```python
from build123d import *

# Parameters (mm, degrees)
EXTRUDE_1_DEPTH                 = 60
SKETCH_3_W                      = 44.3
SKETCH_3_H                      = 33.8
CUT_EXTRUDE_1_DEPTH             = 56.5
SKETCH_4_W                      = 75
SKETCH_4_H                      = 30
EXTRUDE_2_DEPTH                 = 66
SKETCH_5_W                      = 59.221662283
SKETCH_5_H                      = 50
CUT_EXTRUDE_2_DEPTH             = 65
SKETCH_34_W                     = 75
SKETCH_34_H                     = 30
EXTRUDE_5_DEPTH                 = 0.5
HOLE_WIZARD_M3_1_AT_2_COUNT     = 2
HOLE_WIZARD_M3_1_AT_2_PITCH     = 21
HOLE_WIZARD_M3_1_AT_3_COUNT     = 2
HOLE_WIZARD_M3_1_AT_3_PITCH     = 24.186773245
HOLE_WIZARD_M3_1_AT_4_COUNT     = 2
HOLE_WIZARD_M3_1_AT_4_PITCH     = 12
SKETCH_9_W                      = 201.131722391
SKETCH_9_H                      = 182.70094424
CUT_EXTRUDE_3_DEPTH             = 10
SKETCH_10_W                     = 66.5
SKETCH_10_H                     = 50
CUT_EXTRUDE_4_DEPTH             = 1.2
HOLE_WIZARD_M2_5_1_D            = 2.7
HOLE_WIZARD_M2_5_1_CBORE_D      = 5.5
HOLE_WIZARD_M2_5_1_CBORE_DEPTH  = 2.9
EXTRUDE_3_DEPTH                 = 12
SKETCH_16_W                     = 66.5
SKETCH_16_H                     = 53.8
EXTRUDE_4_DEPTH                 = 3
HOLE_WIZARD_M2_5_2_D            = 2.7
HOLE_WIZARD_M2_5_2_DEPTH        = 10
HOLE_WIZARD_M2_5_2_CBORE_D      = 5.5
HOLE_WIZARD_M2_5_2_CBORE_DEPTH  = 5
HOLE_START                      = -61.2
HOLE_WIZARD_2_9_2_9_1_OUTLINE_R = 1.45
HOLE_WIZARD_2_9_2_9_1_DEPTH     = 10
HOLE_START_2                    = -56.2
HOLE_WIZARD_2_9_2_9_2_OUTLINE_R = 1.45
HOLE_WIZARD_2_9_2_9_2_DEPTH     = 5
HOLE_WIZARD_2_9_2_9_4_D         = 2.9
HOLE_WIZARD_2_9_2_9_4_DEPTH     = 7
HOLE_WIZARD_2_9_2_9_4_TIP       = 0.871247898
CUT_EXTRUDE_5_REACH             = 165.928


# Read off the part's stored shape, not the designer's step: Ø2.9 (2.9) 直径孔1, Ø2.9 (2.9) 直径孔2, Ø2.9 (2.9) 直径孔3
with BuildPart() as part:
    # 草图2 → 凸台-拉伸1 (new body)
    with BuildSketch(Plane.XY):
        Polygon((0, 0), (15.232865332, 0), (15.232865332, -50), (66.5, -50), (66.5, -105), (0, -105), align=None)
    extrude(amount=EXTRUDE_1_DEPTH)

    # 草图3 → 切除-拉伸1 (cut)
    with BuildSketch(Plane.ZY):
        with Locations((37.85, -78.1)):
            Rectangle(SKETCH_3_W, SKETCH_3_H)
    extrude(amount=-CUT_EXTRUDE_1_DEPTH, mode=Mode.SUBTRACT)

    # 草图4 → 凸台-拉伸2 (add)
    with BuildSketch(Plane.ZY):
        with Locations((37.5, -120)):
            Rectangle(SKETCH_4_W, SKETCH_4_H)
    extrude(amount=-EXTRUDE_2_DEPTH)

    # 草图5 → 切除-拉伸2 (cut)
    with BuildSketch(Plane.XY.offset(60)):
        with Locations((-14.37796581, -25)):
            Rectangle(SKETCH_5_W, SKETCH_5_H)
    extrude(amount=-CUT_EXTRUDE_2_DEPTH, mode=Mode.SUBTRACT)

    # 草图34 → 凸台-拉伸5 (add)
    with BuildSketch(Plane(origin=(66, 0, 0), x_dir=(0, 0, -1), z_dir=(1, 0, 0))):
        with Locations((-37.5, -120)):
            Rectangle(SKETCH_34_W, SKETCH_34_H)
    extrude(amount=EXTRUDE_5_DEPTH)

    # 草图8 → M3 六角凹头螺钉的柱形沉头孔1 (revolve, cut)
    with BuildSketch(Plane(origin=(66, -108.3, 54.5), x_dir=(0, 0, -1), z_dir=(0, 1, 0))):
        Polygon((0, 0), (0, 66), (1.45, 66), (1.45, 60), (3.25, 60), (3.25, 0), align=None)
    hole_wizard_m3_1 = revolve(axis=Axis((72.35, -108.3, 54.5), (-1, 0, 0)), mode=Mode.SUBTRACT)

    # M3 六角凹头螺钉的柱形沉头孔1 at 2: M3 六角凹头螺钉的柱形沉头孔1 ×2
    with Locations(*[(0, 0, -i * HOLE_WIZARD_M3_1_AT_2_PITCH) for i in range(1, HOLE_WIZARD_M3_1_AT_2_COUNT)]):
        add(hole_wizard_m3_1, mode=Mode.SUBTRACT)

    # M3 六角凹头螺钉的柱形沉头孔1 at 3: M3 六角凹头螺钉的柱形沉头孔1 ×2
    with Locations(*[Vector(0, -0.4961389383568334, -0.8682431421244595) * (i * HOLE_WIZARD_M3_1_AT_3_PITCH) for i in range(1, HOLE_WIZARD_M3_1_AT_3_COUNT)]):
        add(hole_wizard_m3_1, mode=Mode.SUBTRACT)

    # M3 六角凹头螺钉的柱形沉头孔1 at 4: M3 六角凹头螺钉的柱形沉头孔1 ×2
    with Locations(*[(0, -i * HOLE_WIZARD_M3_1_AT_4_PITCH, 0) for i in range(1, HOLE_WIZARD_M3_1_AT_4_COUNT)]):
        add(hole_wizard_m3_1, mode=Mode.SUBTRACT)

    # 草图9 → 切除-拉伸3 (cut)
    with BuildSketch(Plane(origin=(0, 0, 0), x_dir=(-1, 0, 0), z_dir=(0, 0, -1))):
        with Locations((-9.064738267, -112.548341422)):
            Rectangle(SKETCH_9_W, SKETCH_9_H)
    extrude(amount=-CUT_EXTRUDE_3_DEPTH, mode=Mode.SUBTRACT)

    # 草图10 → 切除-拉伸4 (cut)
    with BuildSketch(Plane(origin=(0, -50, 0), x_dir=(1, 0, 0), z_dir=(0, 1, 0))):
        with Locations((33.25, -35)):
            Rectangle(SKETCH_10_W, SKETCH_10_H)
    extrude(amount=-CUT_EXTRUDE_4_DEPTH, mode=Mode.SUBTRACT)

    # M2.5 六角凹头螺钉的柱形沉头孔1 (through all)
    with Locations(Plane(origin=(66.5, 0, 0), x_dir=(0, 0, -1), z_dir=(1, 0, 0))):
        with Locations((-29.85, -68.1), (-45.85, -68.1), (-45.85, -88.1), (-29.85, -88.1)):
            CounterBoreHole(HOLE_WIZARD_M2_5_1_D / 2, HOLE_WIZARD_M2_5_1_CBORE_D / 2, HOLE_WIZARD_M2_5_1_CBORE_DEPTH)

    # 草图15 → 凸台-拉伸3 (add)
    with BuildSketch(Plane.XY.offset(60)):
        Polygon((66.5, -105), (66.5, -51.2), (0, -51.2), (0, -56.2), (46.5, -56.2), (46.5, -100), (0, -100), (0, -105), align=None)
    extrude(amount=EXTRUDE_3_DEPTH)

    # 草图16 → 凸台-拉伸4 (add)
    with BuildSketch(Plane.XY.offset(72)):
        with Locations((33.25, -78.1)):
            Rectangle(SKETCH_16_W, SKETCH_16_H)
    extrude(amount=EXTRUDE_4_DEPTH)

    # M2.5 六角凹头螺钉的柱形沉头孔2
    with Locations(Plane(origin=(0, -51.2, 0), x_dir=(1, 0, 0), z_dir=(0, 1, 0))):
        with Locations((17.75, -45.85), (17.75, -29.85), (49.75, -29.85), (49.75, -45.85)):
            CounterBoreHole(HOLE_WIZARD_M2_5_2_D / 2, HOLE_WIZARD_M2_5_2_CBORE_D / 2, HOLE_WIZARD_M2_5_2_CBORE_DEPTH, depth=HOLE_WIZARD_M2_5_2_DEPTH)

    # Ø2.9 (2.9) 直径孔1 outline → Ø2.9 (2.9) 直径孔1 (cut)
    with BuildSketch(Plane(origin=(0, 0, 0), x_dir=(1, 0, 0), z_dir=(0, 1, 0)).offset(HOLE_START)):
        with Locations((39.499246981, -23.35)):
            Circle(HOLE_WIZARD_2_9_2_9_1_OUTLINE_R)
        with Locations((47.499246981, -36.35)):
            Circle(HOLE_WIZARD_2_9_2_9_1_OUTLINE_R)
        with Locations((47.499246981, -23.35)):
            Circle(HOLE_WIZARD_2_9_2_9_1_OUTLINE_R)
        with Locations((39.499246981, -36.35)):
            Circle(HOLE_WIZARD_2_9_2_9_1_OUTLINE_R)
        with Locations((23.5, -44.6)):
            Circle(HOLE_WIZARD_2_9_2_9_1_OUTLINE_R)
        with Locations((23.5, -15.1)):
            Circle(HOLE_WIZARD_2_9_2_9_1_OUTLINE_R)
        with Locations((6, -23.1)):
            Circle(HOLE_WIZARD_2_9_2_9_1_OUTLINE_R)
        with Locations((6, -36.6)):
            Circle(HOLE_WIZARD_2_9_2_9_1_OUTLINE_R)
    extrude(amount=HOLE_WIZARD_2_9_2_9_1_DEPTH, mode=Mode.SUBTRACT)

    # Ø2.9 (2.9) 直径孔2 outline → Ø2.9 (2.9) 直径孔2 (cut)
    with BuildSketch(Plane(origin=(0, 0, 0), x_dir=(1, 0, 0), z_dir=(0, 1, 0)).offset(HOLE_START_2)):
        with Locations((39.5, -60.3)):
            Circle(HOLE_WIZARD_2_9_2_9_2_OUTLINE_R)
        with Locations((9, -60.3)):
            Circle(HOLE_WIZARD_2_9_2_9_2_OUTLINE_R)
    extrude(amount=HOLE_WIZARD_2_9_2_9_2_DEPTH, mode=Mode.SUBTRACT)

    # Ø2.9 (2.9) 直径孔3 outline → Ø2.9 (2.9) 直径孔3 (revolve, cut)
    with BuildSketch(Plane(origin=(59.999246981, 0, 19.3), x_dir=(1, 0, 0), z_dir=(0, 0, 1))):
        Polygon((0, -51.2), (0, -62.071247898), (1.45, -61.2), (1.45, -51.2), align=None)
    revolve(axis=Axis((59.999246981, 0, 19.3), (0, 1, 0)), mode=Mode.SUBTRACT)

    # Ø2.9 (2.9) 直径孔4
    with Locations(Plane(origin=(0, -135, 0), x_dir=(-1, 0, 0), z_dir=(0, -1, 0))):
        with Locations((-23.5, -15.1), (-39.499246981, -23.35), (-47.499246981, -23.35), (-59.999246981, -19.3), (-47.499246981, -36.35), (-39.499246981, -36.35), (-39.5, -60.3), (-23.5, -44.6), (-6, -36.6), (-6, -23.1), (-9, -60.3)):
            Hole(HOLE_WIZARD_2_9_2_9_4_D / 2, depth=HOLE_WIZARD_2_9_2_9_4_DEPTH)
            with Locations((0, 0, -(HOLE_WIZARD_2_9_2_9_4_DEPTH + HOLE_WIZARD_2_9_2_9_4_TIP / 2))):  # 118° drill point
                Cone(0, HOLE_WIZARD_2_9_2_9_4_D / 2, HOLE_WIZARD_2_9_2_9_4_TIP, mode=Mode.SUBTRACT)

    # 切除-拉伸5: up to this face of the body (flat: up to its plane)
    cut_extrude_5_end = Plane(part.part.faces().sort_by_distance((28.25, -78.1, 15.7))[0])
    # 草图33 → 切除-拉伸5 (cut, up to the picked face)
    with BuildSketch(Plane(origin=(0, 0, 10), x_dir=(-1, 0, 0), z_dir=(0, 0, -1)), mode=Mode.PRIVATE) as cut_extrude_5_sk1:
        Polygon((-21, -61.1), (-37, -61.1), (-34.176470588, -67.1), (-21, -67.1), align=None)
    cut_extrude_5_tool1 = split(extrude(cut_extrude_5_sk1.sketch, amount=-CUT_EXTRUDE_5_REACH, mode=Mode.PRIVATE), bisect_by=cut_extrude_5_end, keep=Keep.BOTH, mode=Mode.PRIVATE)
    # 草图33 → 切除-拉伸5 (cut, up to the picked face)
    with BuildSketch(Plane(origin=(0, 0, 10), x_dir=(-1, 0, 0), z_dir=(0, 0, -1)), mode=Mode.PRIVATE) as cut_extrude_5_sk2:
        Polygon((-23.823529412, -89.1), (-37, -89.1), (-37, -95.1), (-21, -95.1), align=None)
    cut_extrude_5_tool2 = split(extrude(cut_extrude_5_sk2.sketch, amount=-CUT_EXTRUDE_5_REACH, mode=Mode.PRIVATE), bisect_by=cut_extrude_5_end, keep=Keep.BOTH, mode=Mode.PRIVATE)
    # 草图33 → 切除-拉伸5 (cut, up to the picked face)
    with BuildSketch(Plane(origin=(0, 0, 10), x_dir=(-1, 0, 0), z_dir=(0, 0, -1)), mode=Mode.PRIVATE) as cut_extrude_5_sk3:
        Polygon((-21, -89.1), (-23.823529412, -89.1), (-21, -95.1), align=None)
    cut_extrude_5_tool3 = split(extrude(cut_extrude_5_sk3.sketch, amount=-CUT_EXTRUDE_5_REACH, mode=Mode.PRIVATE), bisect_by=cut_extrude_5_end, keep=Keep.BOTH, mode=Mode.PRIVATE)
    # 草图33 → 切除-拉伸5 (cut, up to the picked face)
    with BuildSketch(Plane(origin=(0, 0, 10), x_dir=(-1, 0, 0), z_dir=(0, 0, -1)), mode=Mode.PRIVATE) as cut_extrude_5_sk4:
        Polygon((-34.176470588, -67.1), (-37, -61.1), (-37, -67.1), align=None)
    cut_extrude_5_tool4 = split(extrude(cut_extrude_5_sk4.sketch, amount=-CUT_EXTRUDE_5_REACH, mode=Mode.PRIVATE), bisect_by=cut_extrude_5_end, keep=Keep.BOTH, mode=Mode.PRIVATE)
    add(cut_extrude_5_tool1.solids().sort_by(Axis((28.316888, -64.003226, 10), (0, 0, 1)))[0], mode=Mode.SUBTRACT)
    add(cut_extrude_5_tool2.solids().sort_by(Axis((29.683112, -92.196774, 10), (0, 0, 1)))[0], mode=Mode.SUBTRACT)
    add(cut_extrude_5_tool3.solids().sort_by(Axis((21.941176, -91.1, 10), (0, 0, 1)))[0], mode=Mode.SUBTRACT)
    add(cut_extrude_5_tool4.solids().sort_by(Axis((36.058824, -65.1, 10), (0, 0, 1)))[0], mode=Mode.SUBTRACT)


solid = part.part
```
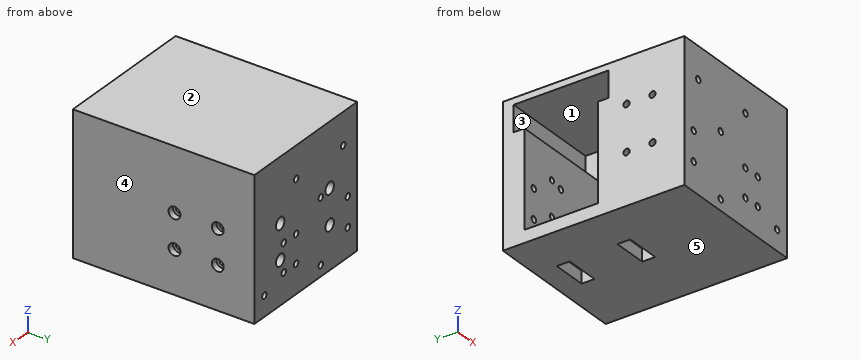
Geometry check sheet. Reference: the model listing, model coordinates, mm. Face numbers are marked on the shaded views. A direction names the side the tool comes from. Coordinates: 2 decimals unless noted, no trailing zeros. Order: outer loops, then holes, each group sorted by start corner. A loop starts at its lowest first (then second) coordinate and runs counter-clockwise, first axis right, second up. Notation, with made-up numbers: (86.5, 33) - (130.5, 33) arc R21 cw to (130.5, 38) - close; hole circle Ø6 at (76.5, -4). An arc over 180 degrees is marked (long way). Use one line per item in the form item = value.
1. Section check A-A (x = 17.75). State how many separate pieces and enclosed holes the cut face has, then the cut area to 3 significant figures.
Here are the results:
separate_pieces = 2
enclosed_holes = 4
area = 3,210 mm²
2. Access from +Z, -Z, +X, -X, +Y, -Y to the whole of each face (thin tool, end or side, straight path). Record for the marked faces 1 and 2.
Here are the results:
face_1 = -X
face_2 = +Z, +X, -X, +Y, -Y
3. Section check D-D (y = -81.5). Record the boundary of the cut face in (x, z), then the cut area to 3 significant figures.
Here are the results:
outline = (0, 10) - (66.5, 10) - (66.5, 75) - (0, 75) - (0, 72) - (46.5, 72) - (46.5, 60) - (56.5, 60) - (56.5, 15.7) - (0, 15.7) - close
area = 1,260 mm²
4. Section check B-B (y = -92.5). Record the boundary of the cut face in (x, z), then the cut area to 3 significant figures.
Here are the results:
outline = (0, 10) - (21, 10) - (21, 15.7) - (0, 15.7) - close; (0, 72) - (46.5, 72) - (46.5, 60) - (56.5, 60) - (56.5, 15.7) - (37, 15.7) - (37, 10) - (66.5, 10) - (66.5, 75) - (0, 75) - close
area = 1,170 mm²
5. Draft check along Z on the marked faces 3, 4 and 5. Enter one of: pulls with the +Z half, pulls with the -Z half, needs draft (parallel to the pull), parting line crosses it, or undercut.
Here are the results:
face_3 = undercut
face_4 = needs draft
face_5 = pulls with the -Z half
6. Scan lines: line 1 (Z direction, x = 6, y = -54); line 2 (Z direction, x = 49.75, y = -59.15); line 3 (X direction, y = -58.25, z = 36.35). Record each from-to range of solid material in increasing order.
Here are the results:
line_1 = 10 to 21.65, 24.55 to 35.15, 38.05 to 75
line_2 = 10 to 28.5, 31.2 to 44.5, 47.2 to 75
line_3 = 0 to 4.57, 7.43 to 38.05, 40.95 to 46.05, 48.95 to 66.5
7. Gauge pin test, flat ends, axial feed: pin 1 (3.5 mm diameter, centred on y = -88.1, z = 29.85, fed in from +X); pin 2 (4.5 mm diameter, centred on x = 49.75, z = 29.85, fed in from +Y); pin 3 (8 mm diameter, centred on y = -73.5, z = 52, fed in from -X). Record the tip position at first contact, or that the pin passes through.
Here are the results:
pin_1 = 63.6
pin_2 = -56.2
pin_3 = 56.5
8. Section check C-C (z = 69.5). Record the boundary of the cut face in (x, y), then the cut area to 3 significant figures.
Here are the results:
outline = (0, -135) - (66.5, -135) - (66.5, -51.2) - (0, -51.2) - (0, -56.2) - (46.5, -56.2) - (46.5, -100) - (0, -100) - close
area = 3,540 mm²
